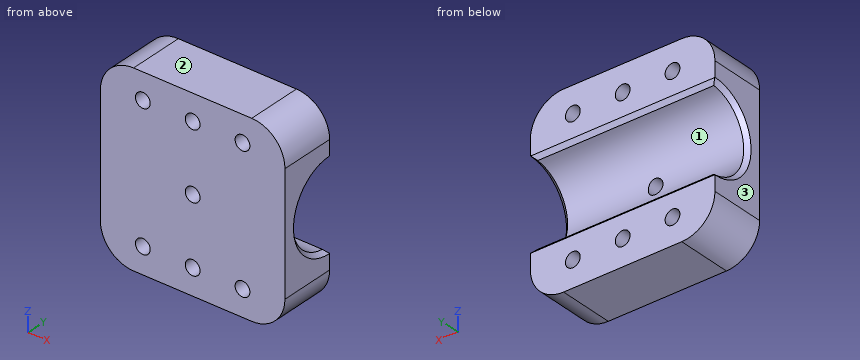
```python
from build123d import *

# Parameters (mm, degrees)
BOSS_EXTRUDE1_DEPTH = 50
SKETCH2_R           = 2
CUT_EXTRUDE1_DEPTH  = 73.582262985
CHAMFER2_START      = -1
CHAMFER2_2_DEPTH    = 52
FILLET3_R           = 9


with BuildPart() as part:
    # Sketch1 → Boss-Extrude1 (new body)
    with BuildSketch(Plane(origin=(0, 0, 0), x_dir=(0, 0, -1), z_dir=(1, 0, 0))):
        with BuildLine():
            Line((14.14, 0), (0, 0))
            Line((0, 0), (0, -15))
            Line((0, -15), (50.43, -15))
            Line((50.43, -15), (50.43, 0))
            Line((50.43, 0), (36.29, 0))
            ThreePointArc((36.29, 0), (25.215, -11.075), (14.14, 0))
        make_face()
    extrude(amount=BOSS_EXTRUDE1_DEPTH)

    # Sketch2 → Cut-Extrude1 (cut, through all)
    with BuildSketch(Plane(origin=(0, 0, 0), x_dir=(1, 0, 0), z_dir=(0, 1, 0))):
        with Locations(Location((11.5, 43.36, 0), (0, 0, 270))):
            Circle(SKETCH2_R)
        with Locations(Location((38.5, 43.36, 0), (0, 0, 90))):
            Circle(SKETCH2_R)
        with Locations(Location((38.5, 7.07, 0), (0, 0, 270))):
            Circle(SKETCH2_R)
        with Locations(Location((11.5, 7.07, 0), (0, 0, 90))):
            Circle(SKETCH2_R)
        with Locations(Location((25, 25.215, 0), (0, 0, 270))):
            Circle(SKETCH2_R)
        with Locations(Location((25, 43.36, 0), (0, 0, 270))):
            Circle(SKETCH2_R)
        with Locations(Location((25, 7.07, 0), (0, 0, 270))):
            Circle(SKETCH2_R)
    extrude(amount=-CUT_EXTRUDE1_DEPTH, mode=Mode.SUBTRACT)

    # Chamfer2: read off the stored shape, not the designer's step
    # Chamfer2 outline → Chamfer2 (revolve, cut)
    with BuildSketch(Plane.YX.offset(25.215)):
        Polygon((12.129624038, 0), (11.075, 1.149849684), (11.075, 0), align=None)
        Polygon((11.075, 50), (11.075, 48.850150316), (12.129624038, 50), align=None)
    revolve(axis=Axis((0, 0, -25.215), (1, 0, 0)), mode=Mode.SUBTRACT)

    # Chamfer2 2 outline → Chamfer2 2 (cut)
    with BuildSketch(Plane.YZ.offset(CHAMFER2_START)):
        with BuildLine():
            Line((0, -14.14), (0, -13.14))
            Line((0, -13.14), (-1.049874688, -14.189874688))
            ThreePointArc((-1.049874688, -14.189874688), (-0.525529339, -14.152475699), (0, -14.14))
        make_face()
        with BuildLine():
            ThreePointArc((0, -36.29), (-0.525529339, -36.277524301), (-1.049874688, -36.240125312))
            Line((-1.049874688, -36.240125312), (0, -37.29))
            Line((0, -37.29), (0, -36.29))
        make_face()
    extrude(amount=CHAMFER2_2_DEPTH, mode=Mode.SUBTRACT)

    # Fillet3
    fillet3_edges = [part.edges().sort_by_distance(p)[0] for p in [
        (50, -7.5, 0),
        (50, -7.5, -50.43),
        (0, -7.5, -50.43),
        (0, -7.5, 0),
    ]]
    fillet(fillet3_edges, radius=FILLET3_R)


solid = part.part
```
The model under review builds one solid part; all positions refer to its coordinate system, in mm. Face numbers are marked on the shaded views. Give positions to 0.01 mm unless a question says otherwise; leave off trailing zeros. Write each loop counter-clockwise with the first axis right and the second up, starting at its lowest first coordinate (ties: lowest second). Pieces come first, ordered by that corner, then holes. Notation, with made-up numbers: (80.5, 25) -> (127.5, 25) arc R6 ccw to (127.5, 35) -> close; hole circle Ø9 at (-12, 89). An arc over 180 degrees is marked (long way). Put each result on its own line as item: value.
(1) We need section C-C, the plane x = 25. Give the boundary of the cut face in (y, z) (3 decimals), and give its area (3 significant figures).
Results are:
outline: (-15, -50.43) -> (0, -50.43) -> (0, -45.36) -> (-15, -45.36) -> close; (-15, -41.36) -> (0, -41.36) -> (0, -37.29) -> (-1.05, -36.24) arc R11.075 cw to (-10.893, -27.215) -> (-15, -27.215) -> close; (-15, -23.215) -> (-10.893, -23.215) arc R11.075 cw to (-1.05, -14.19) -> (0, -13.14) -> (0, -9.07) -> (-15, -9.07) -> close; (-15, -5.07) -> (0, -5.07) -> (0, 0) -> (-15, 0) -> close
area: 427 mm²
(2) We need section B-B, the plane z = -44.5. Give the boundary of the cut face in (x, y), and give its area (3 significant figures).
Results are:
outline: (0.54, -15) -> (9.86, -15) -> (9.86, 0) -> (0.54, 0) -> close; (13.14, -15) -> (23.36, -15) -> (23.36, 0) -> (13.14, 0) -> close; (26.64, -15) -> (36.86, -15) -> (36.86, 0) -> (26.64, 0) -> close; (40.14, -15) -> (49.46, -15) -> (49.46, 0) -> (40.14, 0) -> close
area: 586 mm²
(3) To check wall thickness, follow probe 1 along Z at (x, y) = (24, -12.75); probe 2 along X at (y, z) = (-4.75, -43.36); probe 3 along Y at (x, z) = (13, -25.5). State the ranges of each line that lie inside material, in increasing order. Write a range as from..to.
Results are:
probe 1: -50.43..-45.09, -41.63..-26.95, -23.48..-8.8, -5.34..0
probe 2: 0.21..9.5, 13.5..23, 27..36.5, 40.5..49.79
probe 3: -15..-11.07
(4) We need section D-D, the plane y = -2.25. State how many separate pieces and enclosed holes the cut face has, and give its area (3 significant figures).
Results are:
separate pieces: 2
enclosed holes: 6
area: 1,290 mm²
(5) The part is to be moulded in two halves that separate along Z. For the marked faces 1, 2 and 3, say which applies: pulls with the +Z half, pulls with the -Z half, needs draft (parallel to the pull), parting line crosses it, or undercut.
Results are:
face 1: undercut
face 2: pulls with the +Z half
face 3: needs draft
(6) We need section A-A, the plane x = 38.5. Give the boundary of the cut face in (y, z) (3 decimals), and give its area (3 significant figures).
Results are:
outline: (-15, -50.43) -> (0, -50.43) -> (0, -45.36) -> (-15, -45.36) -> close; (-15, -41.36) -> (0, -41.36) -> (0, -37.29) -> (-1.05, -36.24) arc R11.075 cw to (-1.05, -14.19) -> (0, -13.14) -> (0, -9.07) -> (-15, -9.07) -> close; (-15, -5.07) -> (0, -5.07) -> (0, 0) -> (-15, 0) -> close
area: 443 mm²
(7) For pin 1 Ø1.5 at (x, z) = (36, -33) entering from +Y; pin 2 Ø3.5 at (x, z) = (25, -25.215) entering from -Y; pin 3 Ø5 at (x, z) = (15.5, -20.5) entering from +Y; pin 4 Ø6 at (y, z) = (-2, -45.5) entering from -X, all flat-tipped, find the tip position at first contact; note any pin that passes through.
Results are:
pin 1: y = -7.06
pin 2: through
pin 3: y = -8.4
pin 4: x = 0.06
